Verification items for the finished model (mm, model axes). Face numbers are marked on the shaded views. A direction names the side the tool comes from. Coordinates: 2 decimals unless noted, no trailing zeros. Order: outer loops, then holes, each group sorted by start corner. A loop starts at its lowest first (then second) coordinate and runs counter-clockwise, first axis right, second up. Notation, with made-up numbers: M 34.5,-34.5 L 78.5,-34.5 A11 ccw 78.5,-18.5 Z; hole C 28,27 d4. An arc over 180 degrees is marked long. Return JSON: item names as keys, results as strings.
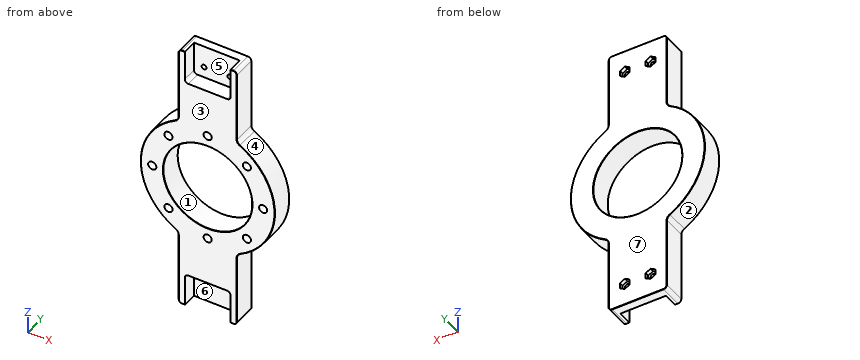
Autodesk Inventor part; units mm, degrees
ref_plane "YZ Plane" through (0, 0, 0) normal (1, 0, 0) x (0, 1, 0)
ref_plane "XZ Plane" through (0, 0, 0) normal (0, 1, 0) x (-1, 0, 0)
ref_plane "XY Plane" through (0, 0, 0) normal (0, 0, 1) x (1, 0, 0)
sketch "Sketch1" plane through (0, 0, 0) normal (0, 1, 0) x (-1, 0, 0)
  circle A0 centre (0, 0) radius 38.125
  line L0 (25, 117.5) -> (-25, 117.5)
  line L1 (-25, -117.5) -> (25, -117.5)
  arc A1 (-25, 51.7808) -> (-25, -51.7808) centre (0, 0) ccw
  arc A2 (25, -51.7808) -> (25, 51.7808) centre (0, 0) ccw
  line L2 (-25, 117.5) -> (-25, 51.7808)
  line L3 (-25, -51.7808) -> (-25, -117.5)
  line L4 (25, -117.5) -> (25, -51.7808)
  line L5 (25, 51.7808) -> (25, 117.5)
  dimension "d0" = 76.25
  dimension "d76" = 50
  dimension "d77" = 57.5
  dimension "d78" = 57.5
  dimension "d79" = 65.7192
  dimension "d80" = 65.7192
  dimension "d81" = 50
  dimension "d82" = 235
extrude "Extrusion1" add sketch "Sketch1" along normal blind 20
fillet "Fillet1" radius 5 4 edges at (-25, 10, 51.7808) (25, 10, 51.7808) (25, 10, -51.7808) (-25, 10, -51.7808)
fillet "Fillet2" radius 3 4 edges at (25, 10, 117.5) (-25, 10, 117.5) (25, 10, -117.5) (-25, 10, -117.5)
chamfer "Chamfer1" distance 0.25 angle 45 26 edges at (25, 20, 84.6646) (57.5, 20, 0) (25, 20, -84.6646) (24.1213, 20, -116.6213) (0, 20, -117.5) (-24.1213, 20, -116.6213) (-25, 20, -84.6646) (-57.5, 20, 0) (-25, 20, 84.6646) (-24.1213, 20, 116.6213) (0, 20, 117.5) (24.1213, 20, 116.6213) (25, 0, 84.6646) (57.5, 0, 0) (25, 0, -84.6646) (24.1213, 0, -116.6213) (0, 0, -117.5) (-24.1213, 0, -116.6213) (-25, 0, -84.6646) (-57.5, 0, 0) (-25, 0, 84.6646) (-24.1213, 0, 116.6213) (0, 0, 117.5) (24.1213, 0, 116.6213) (38.125, 20, 0) (38.125, 0, 0)
sketch "Sketch3" plane through (0, 0, 0) normal (0, -1, 0) x (1, 0, 0)
  line L0 (-22, -117.25) -> (-22, 117.25)
  line L1 (22, 117.25) -> (22, -117.25)
  line L2 (22, -117.25) -> (-22, 117.25) construction
  line L3 (-22, -117.25) -> (22, 117.25) construction
  line L4 (16.625, 89) -> (-16.625, 89)
  line L5 (-19.625, 92) -> (-19.625, 117.25)
  line L6 (19.625, 117.25) -> (19.625, 92)
  line L7 (19.625, 89) -> (17.4099, 92.7868) construction
  line L8 (-19.625, 89) -> (-17.1837, 91.5811) construction
  line L9 (-19.625, -117.25) -> (-19.625, -91.9916)
  line L10 (-16.6334, -88.9916) -> (16.6165, -88.8986)
  line L11 (19.6248, -91.8986) -> (19.6248, -117.25)
  line L12 (-17.2012, -91.6745) -> (-19.625, -89) construction
  line L13 (17.2501, -91.935) -> (19.6248, -88.8902) construction
  line L14 (22, 117.25) -> (19.625, 117.25)
  line L15 (-22, 117.5) -> (22, 117.5)
  line L16 (-19.625, 117.25) -> (-22, 117.25)
  arc A0 (-16.6334, -88.9916) -> (-19.625, -91.9916) centre (-16.625, -91.9916) ccw
  arc A1 (19.6248, -91.8986) -> (16.6165, -88.8986) centre (16.6248, -91.8986) ccw
  arc A2 (-19.625, 92) -> (-16.625, 89) centre (-16.625, 92) ccw
  arc A3 (16.625, 89) -> (19.625, 92) centre (16.625, 92) ccw
  line L17 (19.6248, -117.25) -> (19.6248, -121.1164)
  line L18 (19.6248, -121.1164) -> (-19.625, -121.1164)
  line L19 (-19.625, -121.1164) -> (-19.625, -117.25)
  line L20 (19.625, 117.25) -> (19.625, 123.825)
  line L21 (19.625, 123.825) -> (-19.625, 123.825)
  line L22 (-19.625, 123.825) -> (-19.625, 117.25)
  line L23 (19.625, 117.25) -> (19.6248, 117.25)
  line L24 (22, -117.25) -> (19.6248, -117.25)
  line L25 (-19.625, -117.25) -> (-22, -117.25)
  point P0 (0, 0)
  point P1 (-19.625, 117.5)
  point P2 (19.625, 117.5)
  dimension "d35" = 39.25
  dimension "d37" = 28.25
  dimension "d38" = 28.25
  dimension "d39" = 39.25
  dimension "d40" = 3
  dimension "d41" = 3
  dimension "d42" = 3
  dimension "d50" = 2.375
  dimension "d51" = 2.375
  dimension "d52" = 44
  dimension "d53" = 39.2499
  dimension "d55" = 2.3752
  dimension "d56" = 2.375
  dimension "d83" = 234.5
extrude "Extrusion4" cut sketch "Sketch3" against normal blind 12.575 contours L9 A0 L10 A1 L11 L17 L18 L19 | L22 L15 L20 L6 A3 L4 A2 L5 | L22 L21 L20 L15
sketch "Sketch4" plane through (0, 12.575, 0) normal (0, -1, 0) x (1, 0, 0)
  circle A0 centre (11, 98.5) radius 2.2451
  circle A1 centre (-11, 98.5) radius 2.3292
  circle A2 centre (10.9998, -98.5) radius 1.5784
  circle A3 centre (-11.0002, -98.5) radius 2.3162
  line L0 (19.6248, -117.5) -> (-19.625, -117.5)
  line L1 (-19.625, -117.5) -> (-19.625, -91.9916)
  line L2 (19.6248, -91.8986) -> (19.6248, -117.5)
  line L3 (-19.625, 117.5) -> (19.625, 117.5)
  line L4 (19.625, 117.25) -> (19.625, 92)
  point P0 (0, 0)
  point P1 (-19.625, -117.25)
  point P2 (19.6248, -117.25)
  dimension "d45" = 19
  dimension "d48" = 19
  dimension "d57" = 19
  dimension "d58" = 19
  dimension "d59" = 22
  dimension "d60" = 22
  dimension "d61" = 8.625
  dimension "d62" = 8.625
hole "Hole2" at (11, 12.575, 98.5) at (-11, 12.575, 98.5) at (10.9998, 12.575, -98.5) at (-11.0002, 12.575, -98.5) direction (0, 1, 0) diameter 4.134 end through all
sketch "Sketch5" plane through (0, 20, 0) normal (0, 1, 0) x (1, 0, 0)
  circle A0 centre (-11, -98.5) radius 2.067
  line L0 (-11, -93.7369) -> (-6.875, -96.1184)
  line L1 (-6.875, -96.1184) -> (-6.875, -100.8816)
  line L2 (-6.875, -100.8816) -> (-11, -103.2631)
  line L3 (-11, -103.2631) -> (-15.125, -100.8816)
  line L4 (-15.125, -100.8816) -> (-15.125, -96.1184)
  line L5 (-15.125, -96.1184) -> (-11, -93.7369)
  circle A1 centre (11, -98.5) radius 2.067
  line L6 (11, -93.7369) -> (15.125, -96.1184)
  line L7 (15.125, -96.1184) -> (15.125, -100.8816)
  line L8 (15.125, -100.8816) -> (11, -103.2631)
  line L9 (11, -103.2631) -> (6.875, -100.8816)
  line L10 (6.875, -100.8816) -> (6.875, -96.1184)
  line L11 (6.875, -96.1184) -> (11, -93.7369)
  circle A2 centre (-11.0002, 98.5) radius 2.067
  line L12 (-11.0002, 93.7369) -> (-15.1252, 96.1184)
  line L13 (-15.1252, 96.1184) -> (-15.1252, 100.8816)
  line L14 (-15.1252, 100.8816) -> (-11.0002, 103.2631)
  line L15 (-11.0002, 103.2631) -> (-6.8752, 100.8816)
  line L16 (-6.8752, 100.8816) -> (-6.8752, 96.1184)
  line L17 (-6.8752, 96.1184) -> (-11.0002, 93.7369)
  circle A3 centre (10.9998, 98.5) radius 2.067
  line L18 (10.9998, 103.2631) -> (15.1248, 100.8816)
  line L19 (15.1248, 100.8816) -> (15.1248, 96.1184)
  line L20 (15.1248, 96.1184) -> (10.9998, 93.7369)
  line L21 (10.9998, 93.7369) -> (6.8748, 96.1184)
  line L22 (6.8748, 96.1184) -> (6.8748, 100.8816)
  line L23 (6.8748, 100.8816) -> (10.9998, 103.2631)
  point P0 (0, 0)
  point P1 (-13.0625, -102.0724)
  point P2 (-8.9377, 94.9276)
  dimension "d70" = 8.25
  dimension "d71" = 8.25
  dimension "d72" = 8.25
  dimension "d73" = 8.25
extrude "Extrusion5" cut sketch "Sketch5" against normal blind 3.45
sketch "Sketch6" plane through (0, 0, 0) normal (0, -1, 0) x (1, 0, 0)
  circle A0 centre (0, 0) radius 47.5
  circle A1 centre (0, -47.5) radius 3.5
  circle A2 centre (33.5876, -33.5876) radius 3.5
  circle A3 centre (47.5, 0) radius 3.5
  circle A4 centre (33.5876, 33.5876) radius 3.5
  circle A5 centre (0, 47.5) radius 3.5
  circle A6 centre (-33.5876, 33.5876) radius 3.5
  circle A7 centre (-47.5, 0) radius 3.5
  circle A8 centre (-33.5876, -33.5876) radius 3.5
  dimension "d84" = 95
  dimension "d85" = 7
  dimension "d88" = 360
extrude "Extrusion6" cut sketch "Sketch6" against normal blind 7 contours A0 A3 | A0 A3 | A4 A0 | A0 A4 | A2 A0 | A0 A2 | A5 A0 | A0 A5 | A1 A0 | A0 A1 | A6 A0 | A0 A6 | A8 A0 | A0 A8 | A7 A0 | A0 A7
properties part number "Head Thing"
Q1. Cross-section at C-C, the plane z = -65. Record the boundary of the cut face in (x, y), and give its area (4 significant figures).
Values:
{"outline": "M -25,0.25 L -24.75,0 L 24.75,0 L 25,0.25 L 25,19.75 L 24.75,20 L -24.75,20 L -25,19.75 Z", "area": "1,000 mm^2"}
Q2. Go/stop test with flat-tipped pins: pin 1 (4 mm diameter, centred on x = 0, z = 47.5, fed in from -Y); pin 2 (4 mm diameter, centred on y = 19, z = -98.5, fed in from -X); pin 3 (4 mm diameter, centred on y = 4, z = 104.5, fed in from +X). Record where each tip stops, or that it passes through.
Values:
{"pin 1": "y = 7", "pin 2": "x = -25", "pin 3": "x = 25"}
Q3. Tool access check on the marked faces 5, 6 and 7. Record the directions out of +Z, -Z, +X, -X, +Y, -Y that give a thin tool (end or side, any length) a straight path to the whole face; none if there is none.
Values:
{"face 5": "+Z, -Y", "face 6": "-Z, -Y", "face 7": "+Z, -Z, +X, -X, +Y"}
Q4. Draft check along X on the marked faces 1, 2, 3 and 4. Enter one of: pulls with the +X half, pulls with the -X half, needs draft (parallel to the pull), parting line crosses it, or undercut.
Values:
{"face 1": "undercut", "face 2": "pulls with the -X half", "face 3": "needs draft", "face 4": "pulls with the +X half"}
Q5. Material ranges on line 1 along Z through (x, y) = (0, 5.5) (3 decimals); line 2 along Z through (x, y) = (-10, 17.25); line 3 along X through (y, z) = (17, -91.5), recorded low to high.
Values:
{"line 1": "-88.945 to -51, -44 to -38.125, 38.125 to 44, 51 to 89", "line 2": "-117.5 to -102.69, -94.31 to -36.79, 36.79 to 94.31, 102.69 to 117.5", "line 3": "-25 to 25"}
Q6. Cross-section at A-A, the plane z = 0. Record the boundary of the cut face in (x, y) (3 decimals), and give its area (3 significant figures).
Values:
{"outline": "M -57.5,0.25 L -57.25,0 L -51,0 L -51,7 L -44,7 L -44,0 L -38.375,0 L -38.125,0.25 L -38.125,19.75 L -38.375,20 L -57.25,20 L -57.5,19.75 Z; M 38.125,0.25 L 38.375,0 L 44,0 L 44,7 L 51,7 L 51,0 L 57.25,0 L 57.5,0.25 L 57.5,19.75 L 57.25,20 L 38.375,20 L 38.125,19.75 Z", "area": "677 mm^2"}
Q7. Cross-section at B-B, the plane x = 0. Record the boundary of the cut face in (y, z) (3 decimals).
Values:
{"outline": "M 0,-88.945 L 12.575,-88.945 L 12.575,-117.5 L 19.75,-117.5 L 20,-117.25 L 20,-38.375 L 19.75,-38.125 L 0.25,-38.125 L 0,-38.375 L 0,-44 L 7,-44 L 7,-51 L 0,-51 Z; M 0,38.375 L 0.25,38.125 L 19.75,38.125 L 20,38.375 L 20,117.25 L 19.75,117.5 L 12.575,117.5 L 12.575,89 L 0,89 L 0,51 L 7,51 L 7,44 L 0,44 Z"}
